Check sheet for the modelled part. Datum: model origin and axes. Units: mm. Face numbers are marked on the shaded views. Coordinates: 2 decimals unless noted, no trailing zeros. Loops run counter-clockwise (first coordinate to the right, second up) from the corner with the lowest first, then second, coordinate; pieces in that order, holes last. Notation, with made-up numbers: (-29.75, 39) - (3.25, 39) arc R15 cw to (3.25, 61) - close; hole circle Ø3 at (72, 73). An arc over 180 degrees is marked (long way). Use a Markdown table: item, result. Add a question column.
1) Sectioned sample at B-B, the plane z = -53.5. Enter the section's corners in (x, y), then the cut area to 3 significant figures.
2) Go/stop test with flat-tipped pins: P1, Ø4, axis at x = -0.47, z = -8.75, coming from the +Y side; P2, Ø4, axis at x = 1, z = -50, coming from the +Y side. Record where each tip stops, or that it passes through.
3) Thickness scan on line 1 (Z direction, x = 0.5, y = 0.5) (3 decimals); line 2 (Z direction, x = 1, y = 1.25) (1 decimal); line 3 (Y direction, x = -3.25, z = -47). Record the ranges inside material, lowest first.
4) Sectioned sample at A-A, the plane x = -1.75. Enter the section's corners in (y, z) (1 decimal).
5) Draft check along Z on the marked faces 1, 2 and 3. Enter one of: pulls with the +Z half, pulls with the -Z half, needs draft (parallel to the pull), parting line crosses it, or undercut.
6) Sectioned sample at C-C, the plane y = 2.75. State how many separate pieces and enclosed holes the cut face has, then the cut area to 3 significant figures.
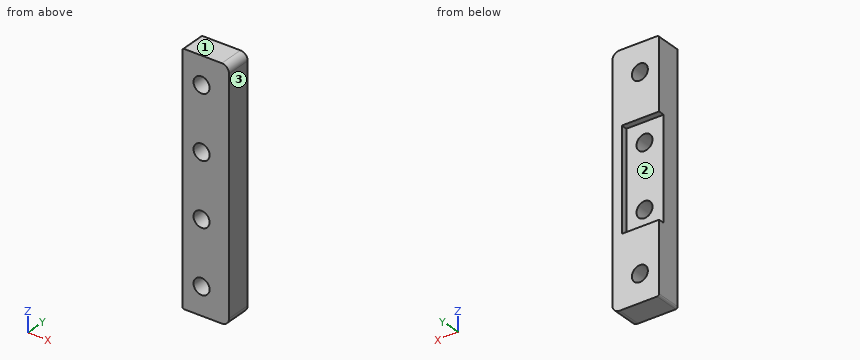
from build123d import *

# Parameters (mm, degrees)
SKETCH1_R           = 2.55
BOSS_EXTRUDE1_DEPTH = 8
SKETCH2_W           = 11.877
SKETCH2_H           = 32.24
CUT_EXTRUDE1_DEPTH  = 2


with BuildPart() as part:
    # Sketch1 → Boss-Extrude1 (new body)
    with BuildSketch(Plane(origin=(0, 0, 0), x_dir=(1, 0, 0), z_dir=(0, 1, 0))):
        with BuildLine():
            Line((-5.97725, 0), (5.97725, 0))
            ThreePointArc((5.97725, 0), (7.615969965, 0.678780035), (8.29475, 2.3175))
            Line((8.29475, 2.3175), (8.29475, 75.1875))
            ThreePointArc((8.29475, 75.1875), (7.615969965, 76.826219965), (5.97725, 77.505))
            Line((5.97725, 77.505), (-5.97725, 77.505))
            ThreePointArc((-5.97725, 77.505), (-6.405049603, 77.327799603), (-6.58225, 76.9))
            Line((-6.58225, 76.9), (-6.58225, 0.605))
            ThreePointArc((-6.58225, 0.605), (-6.405049603, 0.177200397), (-5.97725, 0))
        make_face()
        with Locations((-0.46525, 68.7525)):
            Circle(SKETCH1_R, mode=Mode.SUBTRACT)
        with Locations((-0.46525, 48.7525)):
            Circle(SKETCH1_R, mode=Mode.SUBTRACT)
        with Locations((-0.46525, 8.7525)):
            Circle(SKETCH1_R, mode=Mode.SUBTRACT)
        with Locations((-0.46525, 28.7525)):
            Circle(SKETCH1_R, mode=Mode.SUBTRACT)
    extrude(amount=BOSS_EXTRUDE1_DEPTH)

    # Sketch2 → Cut-Extrude1 (cut)
    with BuildSketch(Plane(origin=(0, 8, 0), x_dir=(1, 0, 0), z_dir=(0, 1, 0))):
        with Locations((-0.64375, 38.7525)):
            Rectangle(SKETCH2_W, SKETCH2_H)
    extrude(amount=-CUT_EXTRUDE1_DEPTH, mode=Mode.SUBTRACT)


solid = part.part
Solved:
| question | item | result |
|---|---|---|
| 1 | outline | (-6.58, 0) - (8.29, 0) - (8.29, 8) - (5.29, 8) - (5.29, 6) - (-6.58, 6) - close |
| 1 | area | 95.3 mm2 |
| 2 | P1 | passes through |
| 2 | P2 | stops at y = 6 |
| 3 | line 1 | z = -77.505 to -71.113, -66.392 to -51.113, -46.392 to -31.113, -26.392 to -11.113, -6.392 to 0 |
| 3 | line 2 | z = -77.5 to -70.8, -66.7 to -50.8, -46.7 to -30.8, -26.7 to -10.8, -6.7 to 0 |
| 3 | line 3 | y = 0 to 6 |
| 4 | outline | (0, -77.5) - (8, -77.5) - (8, -71) - (0, -71) - close; (0, -66.5) - (8, -66.5) - (8, -54.9) - (6, -54.9) - (6, -51) - (0, -51) - close; (0, -46.5) - (6, -46.5) - (6, -31) - (0, -31) - close; (0, -26.5) - (6, -26.5) - (6, -22.6) - (8, -22.6) - (8, -11) - (0, -11) - close; (0, -6.5) - (8, -6.5) - (8, 0) - (0, 0) - close |
| 5 | face 1 | pulls with the +Z half |
| 5 | face 2 | undercut |
| 5 | face 3 | needs draft |
| 6 | separate pieces | 1 |
| 6 | enclosed holes | 4 |
| 6 | area | 1,070 mm2 |
